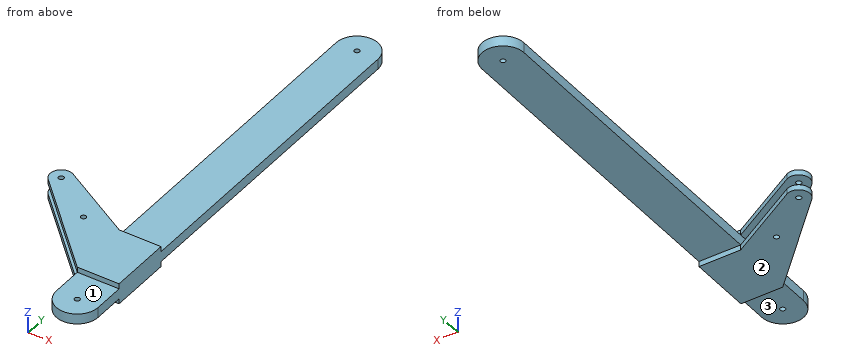
```python
from build123d import *

# Parameters (mm, degrees)
SKETCH1_R           = 1.25
BOSS_EXTRUDE2_DEPTH = 2.45
SKETCH4_R           = 1.25
BOSS_EXTRUDE4_DEPTH = 2.5


with BuildPart() as part:
    # Sketch1 → Boss-Extrude2 (new, symmetric)
    with BuildSketch(Plane.XY):
        with BuildLine():
            Line((-10, -100), (-10, 100))
            ThreePointArc((-10, 100), (0, 110), (10, 100))
            Line((10, 100), (10, -100))
            ThreePointArc((10, -100), (0, -110), (-10, -100))
        make_face()
        with Locations((0, 100)):
            Circle(SKETCH1_R, mode=Mode.SUBTRACT)
        with Locations((0, -100)):
            Circle(SKETCH1_R, mode=Mode.SUBTRACT)
    extrude(amount=BOSS_EXTRUDE2_DEPTH, both=True)

    # Sketch4 → Boss-Extrude4 (add)
    with BuildSketch(Plane.XY.offset(2.45)):
        with BuildLine():
            Line((-10, -85), (-52.426406871, -42.573593129))
            ThreePointArc((-52.426406871, -42.573593129), (-52.884926821, -35.577930556), (-46.008961975, -34.210216111))
            Line((-46.008961975, -34.210216111), (-10, -55))
            Line((-10, -55), (10, -55))
            Line((10, -55), (10, -85))
            Line((10, -85), (-10, -85))
        make_face()
        with Locations((-48.667154687, -38.814340944)):
            Circle(SKETCH4_R, mode=Mode.SUBTRACT)
        with Locations((-26.645631723, -55.712049831)):
            Circle(SKETCH4_R, mode=Mode.SUBTRACT)
    boss_extrude4 = extrude(amount=BOSS_EXTRUDE4_DEPTH)

    # Mirror1: Boss-Extrude4 across plane
    add(boss_extrude4.mirror(Plane.XY))


solid = part.part
```
Here's how the part is built. I have some questions about the finished solid (model axes, mm). Face numbers are marked on the shaded views. A direction names the side the tool comes from. Give positions to 0.01 mm unless a question says otherwise; leave off trailing zeros. Write each loop counter-clockwise with the first axis right and the second up, starting at its lowest first coordinate (ties: lowest second). Pieces come first, ordered by that corner, then holes.
(1) On a 3-axis mill with a long thin cutter (end or side, diameter ignored), from which of +Z, -Z, +X, -X, +Y, -Y can I reach the whole of each face in a straight line? I mean the marked faces 1, 2 and 3. Say none if no direction works.
Output values:
face 1: +Z, +X, -X, -Y
face 2: -Z, +X, -X, +Y, -Y
face 3: -Z, +X, -X, -Y
(2) Imagine slicing it at D-D, the plane x = -7.5. Write out the boundary of the cut face in (y, z).
Output values:
outline: (-106.61, -2.45) - (-85, -2.45) - (-85, -4.95) - (-55, -4.95) - (-55, -2.45) - (106.61, -2.45) - (106.61, 2.45) - (-55, 2.45) - (-55, 4.95) - (-85, 4.95) - (-85, 2.45) - (-106.61, 2.45) - close
(3) Imagine slicing it at B-B, the plane y = -78.5. Write out the boundary of the cut face in (x, z).
Output values:
outline: (-16.5, -4.95) - (10, -4.95) - (10, 4.95) - (-16.5, 4.95) - (-16.5, 2.45) - (-10, 2.45) - (-10, -2.45) - (-16.5, -2.45) - close
(4) Will these pins go through, and if not, where does the flat tip stop? pin 1 (1.5 mm diameter, centred on x = 0, y = 100, fed in from -Z); pin 2 (1.2 mm diameter, centred on x = -2, z = 4.5, fed in from -Y); pin 3 (22 mm diameter, centred on x = -5, y = -13.5, fed in from -Z); pin 4 (6 mm diameter, centred on x = -4, y = 8, fed in from +Z).
Output values:
pin 1: passes through
pin 2: stops at y = -85
pin 3: stops at z = -2.45
pin 4: stops at z = 2.45
(5) Imagine slicing it at C-C, the plane x = -20. Write out the boundary of the cut face in (y, z), and give its area (3 significant figures).
Output values:
outline: (-75, -4.95) - (-49.23, -4.95) - (-49.23, -2.45) - (-75, -2.45) - close; (-75, 2.45) - (-49.23, 2.45) - (-49.23, 4.95) - (-75, 4.95) - close
area: 129 mm2
(6) If I drill on L1, parallel to Y at x = 0, z = -1.75; L2, parallel to X at y = -100, z = 1.4; L3, parallel to Z at x = -29, y = -59, over which ranges is the centre line in solid material (lowest first)?
Output values:
L1: y = -110 to -101.25, -98.75 to 98.75, 101.25 to 110
L2: x = -10 to -1.25, 1.25 to 10
L3: z = -4.95 to -2.45, 2.45 to 4.95
(7) Imagine slicing it at A-A, the plane z = -0.75. Write out the boundary of the cut face in (x, y), and give its area (3 significant figures).
Output values:
outline: (-10, -100) arc R10 ccw to (10, -100) - (10, 100) arc R10 ccw to (-10, 100) - close; hole circle Ø2.5 at (0, -100); hole circle Ø2.5 at (0, 100)
area: 4,300 mm2
